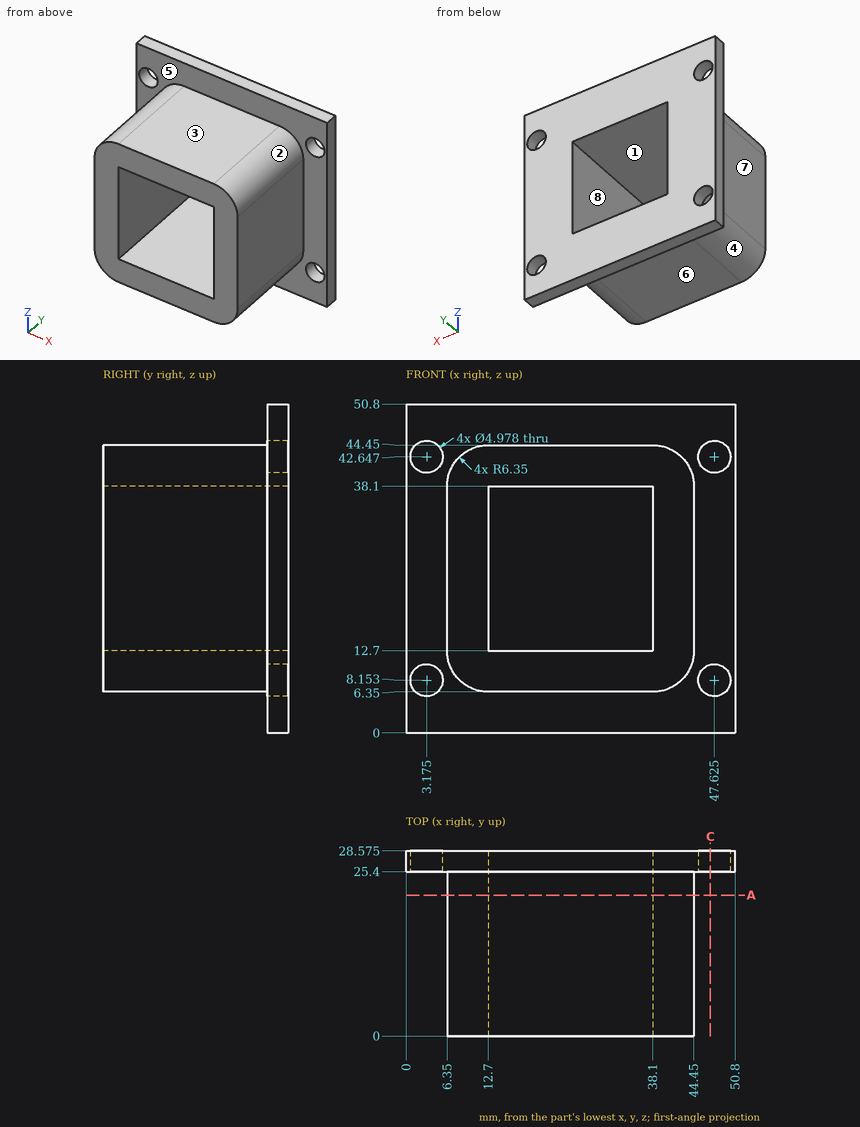
The drawing under review shows one solid part. Ordinate dimensions are in mm from its lowest x, y, z. A direction names the side the tool comes from. Give positions to 0.01 mm unless a question says otherwise; leave off trailing zeros. Order: outer loops, then holes, each group sorted by start corner. A loop starts at its lowest first (then second) coordinate and runs counter-clockwise, first axis right, second up. Notation, with made-up numbers: (0.5, -36.5) -> (38.5, -36.5) arc R20 cw to (38.5, -19.5) -> close; hole circle Ø6 at (39.25, 38.5). An arc over 180 degrees is marked (long way). Write item = value, one per line. Start each with the question number.
(1) For the marked faces 1, 2, 3, 4 and 5, list the 3-axis set-ups (+Z, -Z, +X, -X, +Y, -Y) from which the entire face can be reached by the end or side of a thin tool; tool diameter is ignored.
(2) Mouldability with a two-part tool opening along Z and no side actions: class the marked faces 6, 7 and 8 as +Z half, -Z half, draft (parallel to the pull), parting line (faces both ways), or undercut.
(3) For pin 1 (6 mm diameter, centred on x = 33, y = 16, fed in from +Z); pin 2 (3 mm diameter, centred on y = 21.5, z = 14, fed in from +X); pin 3 (8 mm diameter, centred on x = 3.17, z = 8.15, fed in from -Y); pin 4 (10 mm diameter, centred on x = 20.5, y = 20.5, fed in from -Z), all flat-tipped, find the tip position at first contact; note any pin that passes through.
(4) We need section A-A on y = 21.75. Write out the cut boundary in (x, z).
(5) We need section C-C on x = 47. Write out the cut boundary in (y, z) (1 decimal).
(6) To check wall thickness, follow line 1 along Z through (x, y) = (27.5, 1); line 2 along Y through (x, z) = (42, 5.5) (1 decimal). State the ranges of each line that lie inside material, in increasing order.
Numbers:
q1.face_1 = +Y, -Y
q1.face_2 = +Z, +X, -Y
q1.face_3 = +Z, +X, -X, -Y
q1.face_4 = -Z, -X, -Y
q1.face_5 = -Y
q2.face_6 = -Z half
q2.face_7 = draft
q2.face_8 = undercut
q3.pin_1 = 44.45
q3.pin_2 = 44.45
q3.pin_3 = 25.4
q3.pin_4 = 0
q4.outline = (6.35, 12.7) arc R6.35 ccw to (12.7, 6.35) -> (38.1, 6.35) arc R6.35 ccw to (44.45, 12.7) -> (44.45, 38.1) arc R6.35 ccw to (38.1, 44.45) -> (12.7, 44.45) arc R6.35 ccw to (6.35, 38.1) -> close; hole (12.7, 12.7) -> (38.1, 12.7) -> (38.1, 38.1) -> (12.7, 38.1) -> close
q5.outline = (25.4, 0) -> (28.6, 0) -> (28.6, 5.7) -> (25.4, 5.7) -> close; (25.4, 10.6) -> (28.6, 10.6) -> (28.6, 40.2) -> (25.4, 40.2) -> close; (25.4, 45.1) -> (28.6, 45.1) -> (28.6, 50.8) -> (25.4, 50.8) -> close
q6.line_1 = 6.35 to 12.7, 38.1 to 44.45
q6.line_2 = 25.4 to 28.6
